Check sheet for the modelled part. Datum: model origin and axes. Units: mm. Face numbers are marked on the shaded views. A direction names the side the tool comes from. Round coordinates to 2 decimals unless told otherwise and drop trailing zeros. Write each loop counter-clockwise with the first axis right and the second up, starting at its lowest first coordinate (ties: lowest second). Pieces come first, ordered by that corner, then holes. Notation, with made-up numbers: (70, -0.75) - (126, -0.75) arc R11 cw to (126, 15.25) - close; hole circle Ø1 at (3.5, 40.5). An arc over 180 degrees is marked (long way). Use one line per item in the form item = value. Start each with the question number.
1) Gauge pin test, flat ends, axial feed: P1, Ø2.5, axis at x = -14.5, y = -15.5, coming from the -Z side; P2, Ø8, axis at x = -9.5, y = -4, coming from the +Z side; P3, Ø4.5, axis at x = 2, y = 8.5, coming from the +Z side. Record the tip position at first contact, or that the pin passes through.
2) Draft check along X on the marked faces 1, 2 and 3. Enter one of: +X half, -X half, draft (parallel to the pull), parting line (faces both ways), or undercut.
3) Section check A-A (y = 5.54). Record the boundary of the cut face in (x, z), then the cut area to 3 significant figures.
4) Section check D-D (x = 0). Record the boundary of the cut face in (y, z), then the cut area to 3 significant figures.
5) Scan lines: probe 1 along Z at (x, y) = (1, -4.5); probe 2 along Y at (x, z) = (0, -3.55); probe 3 along Y at (x, z) = (-6, 1.25). Record each from-to range of solid material in increasing order.
6) Set-up check for the marked faces 4, 5 and 6: record each of +Z, -Z, +X, -X, +Y, -Y from which the full face is reachable in a straight line by a thin tool's end or side.
7) Section check B-B (x = -15). Record the boundary of the cut face in (y, z).
8) Section check C-C (z = 1.25). Record the boundary of the cut face in (x, y), then the cut area to 3 significant figures.
from build123d import *

# Parameters (mm, degrees)
BOSS_EXTRUDE1_DEPTH = 4
BOSS_EXTRUDE2_DEPTH = 2
BOSS_EXTRUDE2_DRAFT = 45
BOSS_EXTRUDE3_DEPTH = 5.5
SKETCH6_R           = 4
CUT_EXTRUDE1_DEPTH  = 18.5
SKETCH7_R           = 6.8
CUT_EXTRUDE2_DEPTH  = 5.4
SKETCH8_R           = 7.8
CUT_EXTRUDE3_DEPTH  = 1.5
SKETCH9_R           = 2.05
CUT_EXTRUDE4_DEPTH  = 15.5
SKETCH10_R          = 4
CUT_EXTRUDE5_DEPTH  = 2
SKETCH11_R          = 4
CUT_EXTRUDE6_DEPTH  = 2
CHAMFER4_SIZE       = 3.5


with BuildPart() as part:
    # Sketch1 → Boss-Extrude1 (new body)
    with BuildSketch(Plane.XY):
        Polygon((7, 15.536167626), (-7, 15.536167626), (-12, 9.536492635), (-12, -2.463507365), (-21.005602907, -11.463832374), (-21.005602907, -17.463832374), (-18.009338566, -20.463832374), (14.990661434, -20.463832374), (32.996264341, -12.45977287), (35.994397093, -9.461640117), (35.994397093, -3.461640117), (32.998132752, -0.461640117), (14.998132752, -0.461640117), (12, 2.536492635), (12, 9.536492635), align=None)
    extrude(amount=-BOSS_EXTRUDE1_DEPTH)


with BuildPart() as boss_extrude2_tool:
    # Sketch2 → Boss-Extrude2 (with draft: the straight prism first)
    with BuildSketch(Plane.XY):
        Polygon((7, 15.536167626), (-7, 15.536167626), (-12, 9.536492635), (-12, -2.463507365), (-21.005602907, -11.463832374), (-21.005602907, -17.463832374), (-18.009338566, -20.463832374), (14.990661434, -20.463832374), (32.996264341, -12.45977287), (35.994397093, -9.461640117), (35.994397093, -3.461640117), (32.998132752, -0.461640117), (14.998132752, -0.461640117), (12, 2.536492635), (12, 9.536492635), align=None)
    extrude(amount=BOSS_EXTRUDE2_DEPTH)
    # Boss-Extrude2: the draft: its side faces are tilted about the plane it starts from
    boss_extrude2_sides = [boss_extrude2_tool.faces().sort_by_distance(p)[0] for p in [
        (0, 15.536167626, 1),
        (-9.5, 12.536330131, 1),
        (-12, 3.536492635, 1),
        (-16.502801453, -6.963669869, 1),
        (-21.005602907, -14.463832374, 1),
        (-19.507470737, -18.963832374, 1),
        (-1.509338566, -20.463832374, 1),
        (23.993462887, -16.461802622, 1),
        (34.495330717, -10.960706493, 1),
        (35.994397093, -6.461640117, 1),
        (34.496264923, -1.961640117, 1),
        (23.998132752, -0.461640117, 1),
        (13.499066376, 1.037426259, 1),
        (12, 6.036492635, 1),
        (9.5, 12.536330131, 1),
    ]]
    draft(boss_extrude2_sides, Plane.XY, BOSS_EXTRUDE2_DRAFT)


with BuildPart() as part_1:
    add(part.part)

    # Boss-Extrude2: add boss_extrude2_tool
    add(boss_extrude2_tool.part)

    # Sketch4 → Boss-Extrude3 (add)
    with BuildSketch(Plane.XY):
        Polygon((32.996264341, -12.45977287), (20.826264341, -12.45977287), (17.996264341, -10.45977287), (17.996264341, -2.45977287), (18.828132752, -0.461640117), (32.998132752, -0.461640117), (35.994397093, -3.461640117), (35.994397093, -9.461640117), align=None)
    extrude(amount=BOSS_EXTRUDE3_DEPTH)

    # Sketch6 → Cut-Extrude1 (cut)
    with BuildSketch(Plane(origin=(0, 0, -4), x_dir=(-1, 0, 0), z_dir=(0, 0, -1))):
        with Locations((0, 5.54)):
            Circle(SKETCH6_R)
    extrude(amount=-CUT_EXTRUDE1_DEPTH, mode=Mode.SUBTRACT)

    # Sketch7 → Cut-Extrude2 (cut)
    with BuildSketch(Plane.XY.offset(2)):
        with Locations((0, 5.54)):
            Circle(SKETCH7_R)
    extrude(amount=-CUT_EXTRUDE2_DEPTH, mode=Mode.SUBTRACT)

    # Sketch8 → Cut-Extrude3 (cut)
    with BuildSketch(Plane.XY.offset(2)):
        with Locations((0, 5.54)):
            Circle(SKETCH8_R)
    extrude(amount=-CUT_EXTRUDE3_DEPTH, mode=Mode.SUBTRACT)

    # Sketch9 → Cut-Extrude4 (cut)
    with BuildSketch(Plane.XY.offset(5.5)):
        with Locations((-15, -14.46)):
            Circle(SKETCH9_R)
        with Locations((30, -6.46)):
            Circle(SKETCH9_R)
    extrude(amount=-CUT_EXTRUDE4_DEPTH, mode=Mode.SUBTRACT)

    # Sketch10 → Cut-Extrude5 (cut)
    with BuildSketch(Plane(origin=(0, 0, -4), x_dir=(-1, 0, 0), z_dir=(0, 0, -1))):
        with Locations((15, -14.46)):
            Circle(SKETCH10_R)
    extrude(amount=-CUT_EXTRUDE5_DEPTH, mode=Mode.SUBTRACT)

    # Sketch11 → Cut-Extrude6 (cut)
    with BuildSketch(Plane(origin=(0, 0, -4), x_dir=(-1, 0, 0), z_dir=(0, 0, -1))):
        with Locations((-30, -6.46)):
            Circle(SKETCH11_R)
    extrude(amount=-CUT_EXTRUDE6_DEPTH, mode=Mode.SUBTRACT)

    # Chamfer4
    chamfer4_edges = [part_1.edges().sort_by_distance(p)[0] for p in [
        (19.411264341, -11.45977287, 5.5),
        (18.412198547, -1.460706493, 5.5),
        (17.996264341, -6.45977287, 5.5),
    ]]
    chamfer(chamfer4_edges, length=CHAMFER4_SIZE - 0.0001)  # a hair under: the kernel refuses the full size


solid = part_1.part
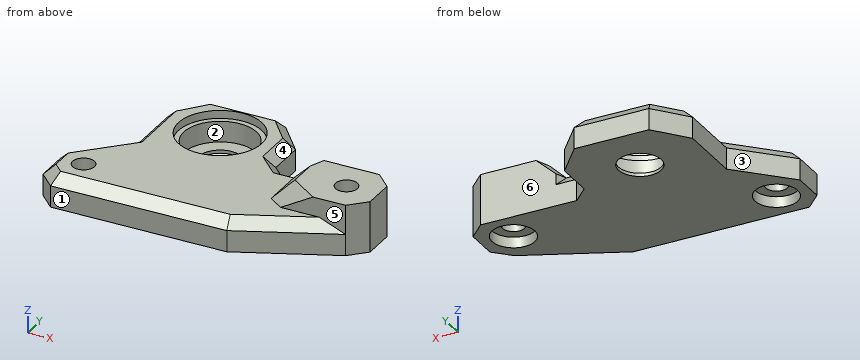
Results are:
q1.P1 = -2
q1.P2 = 2
q1.P3 = -3.4
q2.face_1 = draft
q2.face_2 = undercut
q2.face_3 = -X half
q3.outline = (-12, -4) - (-4, -4) - (-4, -3.4) - (-6.8, -3.4) - (-6.8, 0.5) - (-7.8, 0.5) - (-7.8, 2) - (-10, 2) - (-12, 0) - close; (4, -4) - (12, -4) - (12, 0) - (10, 2) - (7.8, 2) - (7.8, 0.5) - (6.8, 0.5) - (6.8, -3.4) - (4, -3.4) - close
q3.area = 58.8 mm²
q4.outline = (-20.46, -4) - (1.54, -4) - (1.54, -3.4) - (-1.26, -3.4) - (-1.26, 0.5) - (-2.26, 0.5) - (-2.26, 2) - (-18.46, 2) - (-20.46, 0) - close; (9.54, -4) - (15.54, -4) - (15.54, 0) - (13.54, 2) - (13.34, 2) - (13.34, 0.5) - (12.34, 0.5) - (12.34, -3.4) - (9.54, -3.4) - close
q4.area = 131 mm²
q5.probe_1 = -4 to 2
q5.probe_2 = -20.46 to 1.54, 9.54 to 15.54
q5.probe_3 = -19.21 to 0.56, 10.52 to 14.29
q6.face_4 = +Z, +X, +Y
q6.face_5 = +Z, +X, -Y
q6.face_6 = +Z, -Z, +X, +Y
q7.outline = (-20.46, -4) - (-18.46, -4) - (-18.46, -2) - (-16.51, -2) - (-16.51, 2) - (-18.46, 2) - (-20.46, 0) - close; (-12.41, -2) - (-10.46, -2) - (-10.46, -4) - (-5.46, -4) - (-5.46, 0) - (-8.29, 2) - (-12.41, 2) - close
q8.outline = (-19.76, -16.95) - (-17.49, -19.21) - (14.73, -19.21) - (29.92, -12.46) - (33, -12.46) - (35.99, -9.46) - (35.99, -3.46) - (33, -0.46) - (18.83, -0.46) - (18.31, -1.71) - (14.48, -1.71) - (10.75, 2.02) - (10.75, 9.08) - (6.41, 14.29) - (-6.41, 14.29) - (-10.75, 9.08) - (-10.75, -2.98) - (-19.76, -11.98) - close; hole circle Ø4.1 at (-15, -14.46); hole circle Ø15.6 at (0, 5.54); hole circle Ø4.1 at (30, -6.46)
q8.area = 952 mm²
